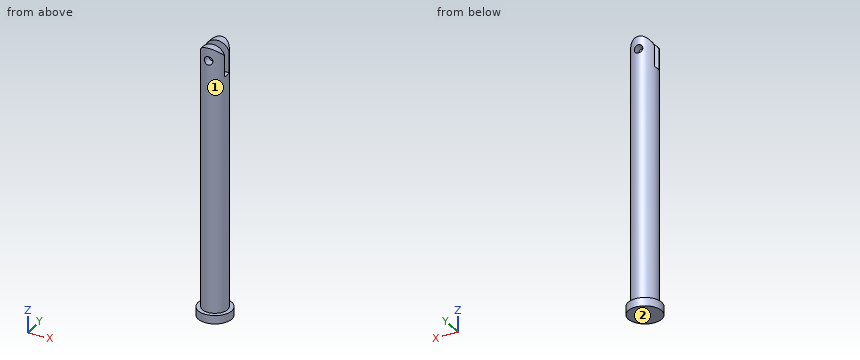
```python
from build123d import *

# Parameters (mm, degrees)
F0_R          = 4.7625
F1_DEPTH      = 101.6
F2_W          = 9.525
F2_H          = 3.175
F3_DEPTH      = 12.7
F4_R          = 1.5875
F5_DEPTH      = 151
F5_DEPTH_BACK = 151
F6_R          = 6.35
F7_DEPTH      = 3.175


# Not quite as in the source:
# - an extrude ends at something that could not be found from the text; its depth is read off the source's solid


with BuildPart() as f1:
    # F0 (on Top) → F1 (new body)
    with BuildSketch(Plane.XY):
        Circle(F0_R)
    extrude(amount=F1_DEPTH)

    # F2 (on face) → F3 (cut)
    with BuildSketch(Plane.XY.offset(101.6)):
        Rectangle(F2_W, F2_H)
    extrude(amount=-F3_DEPTH, mode=Mode.SUBTRACT)

    # F4 (on Front) → F5 (cut, two sides)
    with BuildSketch(Plane.XZ) as f5_sk:
        with BuildLine():
            Line((4.7625, 101.6), (-4.7625, 101.6))
            Line((-4.7625, 101.6), (-4.7625, 95.25))
            ThreePointArc((-4.7625, 95.25), (0, 100.0125), (4.7625, 95.25))
            Line((4.7625, 95.25), (4.7625, 101.6))
        make_face()
        with Locations((0, 95.25)):
            Circle(F4_R)
    extrude(amount=-F5_DEPTH, mode=Mode.SUBTRACT)
    extrude(f5_sk.sketch, amount=F5_DEPTH_BACK, mode=Mode.SUBTRACT)

    # F6 (on face) → F7 (join)
    with BuildSketch(Plane(origin=(0, 0, 0), x_dir=(1, 0, 0), z_dir=(0, 0, -1))):
        Circle(F6_R)
    extrude(amount=F7_DEPTH)


solid = f1.part
```
For this review, take the finished solid that the model builds, in its own axes (mm). Face numbers are marked on the shaded views. A direction names the side the tool comes from. Give positions to 0.01 mm unless a question says otherwise; leave off trailing zeros. Order: outer loops, then holes, each group sorted by start corner. A loop starts at its lowest first (then second) coordinate and runs counter-clockwise, first axis right, second up.
1) Take a section at D-D (z = 43.5). Give the boundary of the cut face in (x, y) (1 decimal), then the cut area to 3 significant figures.
2) Take a section at A-A (x = 0). State how many separate pieces and enclosed holes the cut face has, then the cut area to 4 significant figures.
3) Insertion check: pin 1 (5 mm diameter, centred on x = 0, z = 95.25, fed in from -Y); pin 2 (6 mm diameter, centred on y = -5, z = 45, fed in from -X); pin 3 (4.5 mm diameter, centred on x = 0, z = 96.5, fed in from +Y); pin 4 (1.9 mm diameter, centred on x = 0, z = 95.25, fed in from -Y). Each pin has a flat end and moves straight along its axis. Give the tip position at first contact, or say it passes through.
4) For the marked faces 1 and 2, list the 3-axis set-ups (+Z, -Z, +X, -X, +Y, -Y) from which the entire face can be reached by the end or side of a thin tool; tool diameter is ignored.
5) Wall thickness on line 1 (Z direction, x = 0, y = -4.05) (1 decimal); line 2 (Y direction, x = 0, z = 35); line 3 (Z direction, x = 2.5, y = -4.5) (3 decimals): over which ranges is each line inside the solid? List them lowest first.
6) Take a section at B-B (z = 95.25). Give the boundary of the cut face in (x, y) (1 decimal), then the cut area to 3 significant figures.
Derived:
1. outline: circle Ø9.5 at (0, 0)
1. area: 71.3 mm2
2. separate pieces: 3
2. enclosed holes: 0
2. area: 937.5 mm2
3. pin 1: stops at y = -4.76
3. pin 2: stops at x = -4.32
3. pin 3: stops at y = 4.76
3. pin 4: passes through
4. face 1: +Z
4. face 2: -Z, +X, -X, +Y, -Y
5. line 1: z = -3.2 to 93.7, 96.8 to 100
5. line 2: y = -4.76 to 4.76
5. line 3: z = -3.175 to 0
6. outline: (-4.5, -1.6) arc R4.8 ccw to (-1.6, -4.5) - (-1.6, -1.6) - close; (-4.5, 1.6) - (-1.6, 1.6) - (-1.6, 4.5) arc R4.8 ccw to start; (1.6, -4.5) arc R4.8 ccw to (4.5, -1.6) - (1.6, -1.6) - close; (1.6, 1.6) - (4.5, 1.6) arc R4.8 ccw to (1.6, 4.5) - close
6. area: 22.0 mm2
